Verification items for the finished model (mm, model axes). Face numbers are marked on the shaded views. A direction names the side the tool comes from. Coordinates: 2 decimals unless noted, no trailing zeros. Loops run counter-clockwise (first coordinate to the right, second up) from the corner with the lowest first, then second, coordinate; pieces in that order, holes last. Notation, with made-up numbers: (54, 83.25) - (108, 83.25) arc R21 ccw to (108, 118.25) - close; hole circle Ø9 at (-36.75, 37). An arc over 180 degrees is marked (long way). One line per item, written item: value. Start each with the question number.
(1) Section check A-A (z = -17.5). Record the boundary of the cut face in (x, y).
(2) Draft check along Y on the marked faces 3, 4 and 5. Enter one of: +Y half, -Y half, draft (parallel to the pull), parting line (faces both ways), or undercut.
(3) Set-up check for the marked faces 1 and 2: record each of +Z, -Z, +X, -X, +Y, -Y from which the full face is reachable in a straight line by a thin tool's end or side.
(4) Section check B-B (x = 14.5). Record the boundary of the cut face in (y, z), plus the area to 3 significant figures.
(5) Gauge pin test, flat ends, axial feed: P1, Ø3, axis at y = -29.5, z = -3, coming from the +X side; P2, Ø13, axis at x = -30, y = -41, coming from the +Z side; P3, Ø1.6, axis at x = -81, z = 0.5, coming from the -Y side; P4, Ø14.5, axis at x = -81.5, y = -1, coming from the -Z side. Record the tip position at first contact, or that the pin passes through.
(6) Thickness scan on probe 1 along Y at (x, z) = (-79, -12); probe 2 along Z at (x, y) = (-41, 38); probe 3 along Y at (x, z) = (-75, -13). Record the ranges inside material, lowest first. Write a range as [from, to].
(7) Section check C-C (y = -4). Record the boundary of the cut face in (x, z), plus the area to 3 significant figures.
(8) Section check D-D (x = -80). Record the boundary of the cut face in (y, z), plus the area to 3 significant figures.
```python
from build123d import *

# Parameters (mm, degrees)
F1_DEPTH = 30
F2_DEPTH = 5
F3_DEPTH = 2


with BuildPart() as f1:
    # F0 (on Top) → F1 (new body)
    with BuildSketch(Plane.XY):
        Polygon((-84.5, 46.8874983338), (-85.329787234, 34.9162221635), (-72.329787234, 34.9162221635), (-71.5, 46.8874983338), align=None)
    extrude(amount=-F1_DEPTH)



with BuildPart() as f1b:
    # F0 (on Top) → F1, piece 2 (new body)
    with BuildSketch(Plane.XY):
        Polygon((71.5, 46.8874983338), (72.329787234, 34.9162221635), (85.329787234, 34.9162221635), (84.5, 46.8874983338), align=None)
    extrude(amount=-F1_DEPTH)


with BuildPart() as f1c:
    # F0 (on Top) → F1, piece 3 (new body)
    with BuildSketch(Plane.XY):
        Polygon((77.170212766, -34.9162221635), (78, -46.8874983338), (91, -46.8874983338), (90.170212766, -34.9162221635), align=None)
    extrude(amount=-F1_DEPTH)


with BuildPart() as f1d:
    # F0 (on Top) → F1, piece 4 (new body)
    with BuildSketch(Plane.XY):
        Polygon((-90.170212766, -34.9162221635), (-91, -46.8874983338), (-78, -46.8874983338), (-77.170212766, -34.9162221635), align=None)
    extrude(amount=-F1_DEPTH)


with BuildPart() as f1_1:
    add(f1.part)

    add(f1b.part)  # F2 merges F1b

    add(f1c.part)  # F2 merges F1c

    add(f1d.part)  # F2 merges F1d
    # F0 (on Top) → F2 (join)
    with BuildSketch(Plane.XY):
        Polygon((-85.6763614932, 29.9162221635), (-89.8236385068, -29.9162221635), (-76.8236385068, -29.9162221635), (-72.6763614932, 29.9162221635), align=None)
        Polygon((-85.329787234, 34.9162221635), (-85.6763614932, 29.9162221635), (-72.6763614932, 29.9162221635), (-72.329787234, 34.9162221635), align=None)
        Polygon((-89.8236385068, -29.9162221635), (-90.170212766, -34.9162221635), (-77.170212766, -34.9162221635), (-76.8236385068, -29.9162221635), align=None)
        Polygon((-77.170212766, -34.9162221635), (-78, -46.8874983338), (-72.988003021, -46.8874983338), (-72.158215787, -34.9162221635), align=None)
        Polygon((-72.158215787, -34.9162221635), (-72.988003021, -46.8874983338), (72.988003021, -46.8874983338), (72.158215787, -34.9162221635), align=None)
        Polygon((72.158215787, -34.9162221635), (72.988003021, -46.8874983338), (78, -46.8874983338), (77.170212766, -34.9162221635), align=None)
        Polygon((76.8236385068, -29.9162221635), (77.170212766, -34.9162221635), (90.170212766, -34.9162221635), (89.8236385068, -29.9162221635), align=None)
        Polygon((72.6763614932, 29.9162221635), (76.8236385068, -29.9162221635), (89.8236385068, -29.9162221635), (85.6763614932, 29.9162221635), align=None)
        Polygon((72.329787234, 34.9162221635), (72.6763614932, 29.9162221635), (85.6763614932, 29.9162221635), (85.329787234, 34.9162221635), align=None)
        Polygon((66.488003021, 46.8874983338), (67.3177902551, 34.9162221635), (72.329787234, 34.9162221635), (71.5, 46.8874983338), align=None)
        Polygon((-66.488003021, 46.8874983338), (-67.3177902551, 34.9162221635), (67.3177902551, 34.9162221635), (66.488003021, 46.8874983338), align=None)
        Polygon((-71.5, 46.8874983338), (-72.329787234, 34.9162221635), (-67.3177902551, 34.9162221635), (-66.488003021, 46.8874983338), align=None)
    extrude(amount=-F2_DEPTH)

    # F0 (on Top) → F3 (join)
    with BuildSketch(Plane.XY):
        Polygon((-85.329787234, 34.9162221635), (-85.6763614932, 29.9162221635), (-72.6763614932, 29.9162221635), (-72.329787234, 34.9162221635), align=None)
        Polygon((-89.8236385068, -29.9162221635), (-90.170212766, -34.9162221635), (-77.170212766, -34.9162221635), (-76.8236385068, -29.9162221635), align=None)
        Polygon((72.329787234, 34.9162221635), (72.6763614932, 29.9162221635), (85.6763614932, 29.9162221635), (85.329787234, 34.9162221635), align=None)
        Polygon((76.8236385068, -29.9162221635), (77.170212766, -34.9162221635), (90.170212766, -34.9162221635), (89.8236385068, -29.9162221635), align=None)
    extrude(amount=F3_DEPTH)


solid = f1_1.part
```
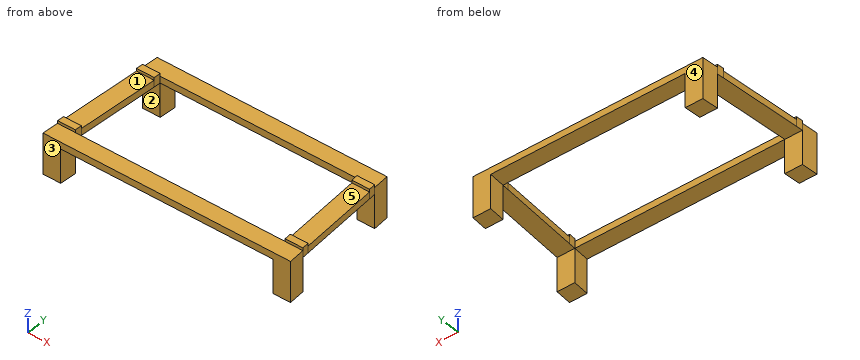
Responses:
1. outline: (-91, -46.89) - (-78, -46.89) - (-77.17, -34.92) - (-90.17, -34.92) - close; (-85.33, 34.92) - (-72.33, 34.92) - (-71.5, 46.89) - (-84.5, 46.89) - close; (71.5, 46.89) - (72.33, 34.92) - (85.33, 34.92) - (84.5, 46.89) - close; (77.17, -34.92) - (78, -46.89) - (91, -46.89) - (90.17, -34.92) - close
2. face 3: -Y half
2. face 4: +Y half
2. face 5: undercut
3. face 1: +Z, +X, -X
3. face 2: -Z, +X, -X
4. outline: (-46.89, -5) - (-34.92, -5) - (-34.92, 0) - (-46.89, 0) - close; (34.92, -5) - (46.89, -5) - (46.89, 0) - (34.92, 0) - close
4. area: 120 mm²
5. P1: stops at x = 89.9
5. P2: stops at z = 0
5. P3: stops at y = -46.89
5. P4: stops at z = -5
6. probe 1: y = [-46.89, -34.92], [34.92, 46.89]
6. probe 2: z = [-5, 0]
6. probe 3: y = [34.92, 46.89]
7. outline: (-88.03, -5) - (-75.03, -5) - (-75.03, 0) - (-88.03, 0) - close; (75.03, -5) - (88.03, -5) - (88.03, 0) - (75.03, 0) - close
7. area: 130 mm²
8. outline: (-46.89, -30) - (-34.92, -30) - (-34.92, -5) - (34.92, -5) - (34.92, -30) - (46.89, -30) - (46.89, 0) - (34.92, 0) - (34.92, 2) - (29.92, 2) - (29.92, 0) - (-29.92, 0) - (-29.92, 2) - (-34.92, 2) - (-34.92, 0) - (-46.89, 0) - close
8. area: 1,090 mm²
